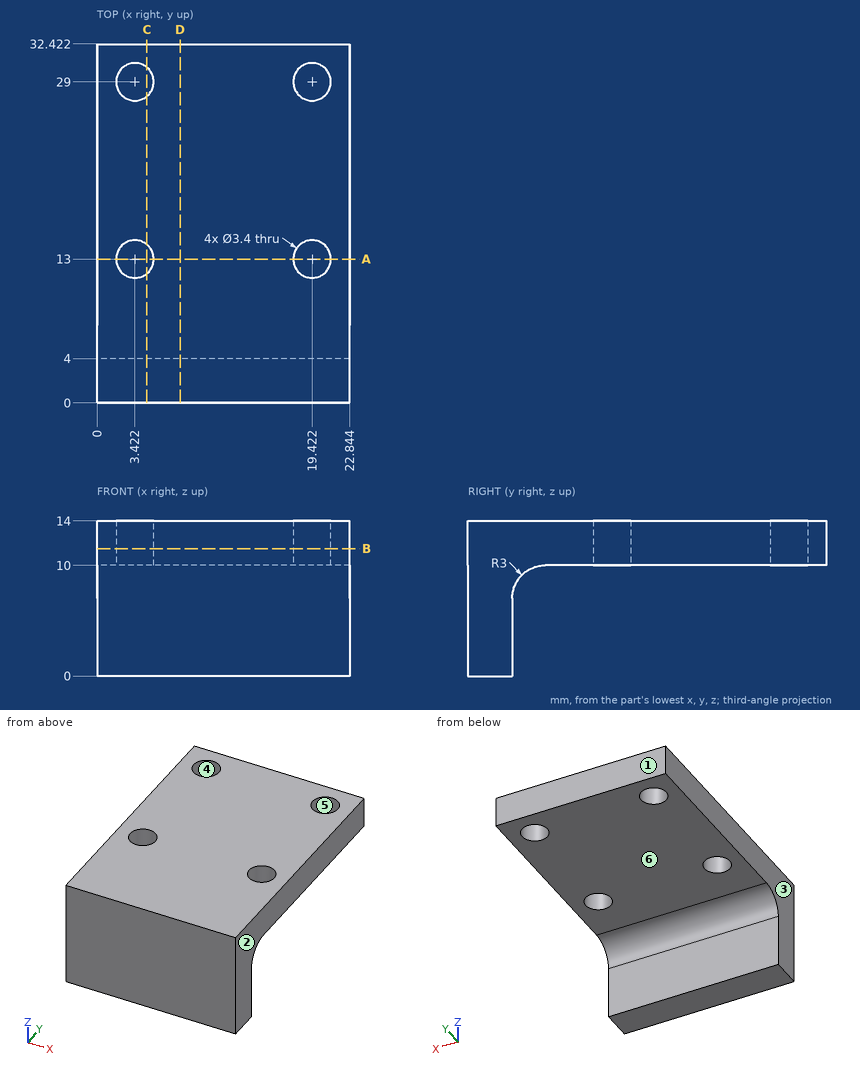
Can you work these out from the drawing? Everything is in mm from the part's minimum corner. A direction names the side the tool comes from. Give positions to 0.01 mm unless a question says otherwise; leave off trailing zeros. Order: outer loops, then holes, each group sorted by start corner. A loop starts at its lowest first (then second) coordinate and runs counter-clockwise, first axis right, second up. Notation, with made-up numbers: (77.25, -26) -> (121.25, -26) arc R17 cw to (121.25, 4) -> close; hole circle Ø11 at (71.25, 70.5). An arc over 180 degrees is marked (long way). Return JSON: item names as keys, results as strings.
1. Imagine slicing it at D-D on x = 7.5. List the corners of the cut face in (y, z) for me.
Answer list:
{"outline": "(0, 0) -> (4, 0) -> (4, 7) arc R3 cw to (7, 10) -> (32.42, 10) -> (32.42, 14) -> (0, 14) -> close"}
2. For pin 1 Ø2 at (x, y) = (3.42, 29) entering from -Z; pin 2 Ø2 at (x, z) = (11, 3.5) entering from +Y; pin 3 Ø4.5 at (x, y) = (19.42, 29) entering from -Z, each with a flat end and sliding along its axis, tell me the tip position at first contact or that it passes through.
Answer list:
{"pin 1": "passes through", "pin 2": "stops at y = 4", "pin 3": "stops at z = 10"}
3. On a 3-axis mill with a long thin cutter (end or side, diameter ignored), from which of +Z, -Z, +X, -X, +Y, -Y can I reach the whole of each face in a straight line? I mean the marked faces 5 and 6. Say none if no direction works.
Answer list:
{"face 5": "+Z, -Z", "face 6": "-Z, +X, -X, +Y"}
4. Imagine slicing it at B-B on z = 11.5. List the corners of the cut face in (x, y) for me.
Answer list:
{"outline": "(0, 0) -> (22.84, 0) -> (22.84, 32.42) -> (0, 32.42) -> close; hole circle Ø3.4 at (3.42, 13); hole circle Ø3.4 at (3.42, 29); hole circle Ø3.4 at (19.42, 13); hole circle Ø3.4 at (19.42, 29)"}
5. Imagine slicing it at C-C on x = 4.5. List the corners of the cut face in (y, z) for me.
Answer list:
{"outline": "(0, 0) -> (4, 0) -> (4, 7) arc R3 cw to (7, 10) -> (11.69, 10) -> (11.69, 14) -> (0, 14) -> close; (14.31, 10) -> (27.69, 10) -> (27.69, 14) -> (14.31, 14) -> close; (30.31, 10) -> (32.42, 10) -> (32.42, 14) -> (30.31, 14) -> close"}
6. Thinking about a two-plate mould opening in X: for the marked faces 1, 2, 3 and 4, which applies, pulls with the +X half, pulls with the -X half, needs draft (parallel to the pull), parting line crosses it, or undercut?
Answer list:
{"face 1": "needs draft", "face 2": "pulls with the +X half", "face 3": "pulls with the -X half", "face 4": "undercut"}
7. I need wall thicknesses on line 1 (Y direction, x = 19.25, z = 11.5); line 2 (Y direction, x = 2.25, z = 11.75); line 3 (Y direction, x = 6.25, z = 5.5). Which ranges of each line are inside material? Lowest first, please. Write a range as from..to.
Answer list:
{"line 1": "y = 0..11.31, 14.69..27.31, 30.69..32.42", "line 2": "y = 0..11.77, 14.23..27.77, 30.23..32.42", "line 3": "y = 0..4"}
8. Imagine slicing it at A-A on y = 13. List the corners of the cut face in (x, z) for me.
Answer list:
{"outline": "(0, 10) -> (1.72, 10) -> (1.72, 14) -> (0, 14) -> close; (5.12, 10) -> (17.72, 10) -> (17.72, 14) -> (5.12, 14) -> close; (21.12, 10) -> (22.84, 10) -> (22.84, 14) -> (21.12, 14) -> close"}
